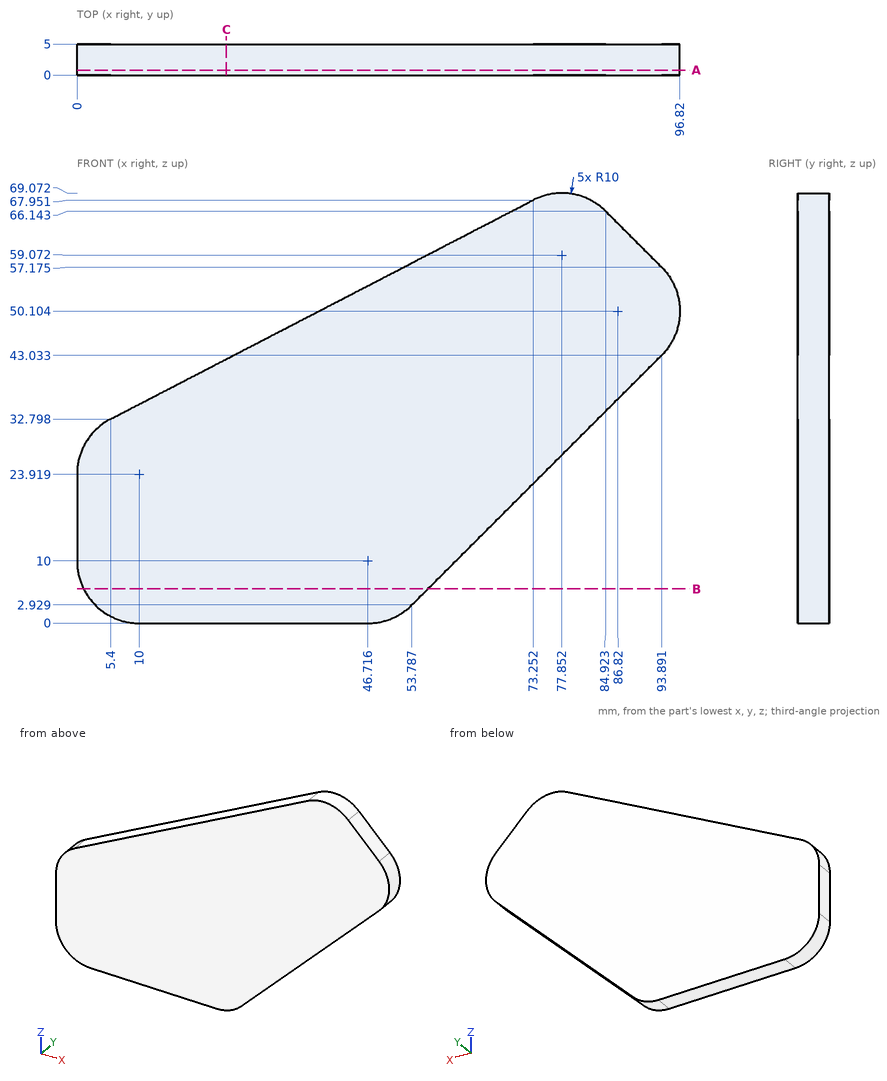
Study the drawing (mm; zero at the part's minimum x, y, z) and answer. Coordinates: 2 decimals unless noted, no trailing zeros. Loops run counter-clockwise (first coordinate to the right, second up) from the corner with the lowest first, then second, coordinate; pieces in that order, holes last. Notation, with made-up numbers: (84, 71.5) -> (137, 71.5) arc R33 cw to (137, 107.5) -> close; hole circle Ø9 at (17, -6). An arc over 180 degrees is marked (long way). Answer in a Markdown table with one row per item. Add a question column.
1. The part is cut by section A-A, the plane y = 0.8. Write down the section's boundary in (x, z) (1 decimal), then the cut area to 3 significant figures.
2. The part is cut by section C-C, the plane x = 24. Write down the section's boundary in (y, z) (1 decimal), then the cut area to 3 significant figures.
3. A flat-ended cylindrical pin translates along its axis: P1, Ø2, axis at y = 2.5, z = 25.5, coming from the -X side. Find the tip coordinate at first contact, or state that the pin passes through.
4. Consider line 1 (Z direction, x = 30.5, y = 0.25); line 2 (X direction, y = 2.2, z = 46) (1 decimal); line 3 (Z direction, x = 70, y = 1.3) (1 decimal). Determine where each line is inside the solid, lowest interval first. Write a range as [from, to].
5. The part is cut by section B-B, the plane z = 5.5. Write down the section's boundary in (x, y).
Answer below:
| question | item | result |
|---|---|---|
| 1 | outline | (0, 10) arc R10 ccw to (10, 0) -> (46.7, 0) arc R10 ccw to (53.8, 2.9) -> (93.9, 43) arc R10 ccw to (93.9, 57.2) -> (84.9, 66.1) arc R10 ccw to (73.3, 68) -> (5.4, 32.8) arc R10 ccw to (0, 23.9) -> close |
| 1 | area | 4,010 mm2 |
| 2 | outline | (0, 0) -> (5, 0) -> (5, 42.4) -> (0, 42.4) -> close |
| 2 | area | 212 mm2 |
| 3 | P1 | x = 0.02 |
| 4 | line 1 | [0, 45.8] |
| 4 | line 2 | [30.9, 95.9] |
| 4 | line 3 | [19.1, 66.3] |
| 5 | outline | (1.07, 0) -> (56.36, 0) -> (56.36, 5) -> (1.07, 5) -> close |
